Autodesk Fusion 360 part; units mm, degrees
sketch "Sketch1" plane through (0, 0, 0) normal (0, 1, 0) x (1, 0, 0)
  line L0 (-7.5, 0) -> (-20, 0)
  line L1 (-20, 0) -> (-20, 8)
  line L2 (-20, 8) -> (20, 8)
  line L3 (20, 8) -> (20, 0)
  line L4 (20, 0) -> (7.5, 0)
  arc A0 (-7.5, 0) -> (7.5, 0) centre (0, 0) ccw
  circle A1 centre (0, 0) radius 4
  dimension "d1" = 15
  dimension "d2" = 20
  dimension "d3" = 20
  dimension "d4" = 8
  dimension "d5" = 8
extrude "Extrude1" add sketch "Sketch1" along normal blind 30 contours L0 L1 L2 L3 L4 A0 | A1
extrude "Extrude2" cut sketch "Sketch1" along normal blind 15 contours A1
fillet "Fillet1" radius 3 4 edges at (-7.5, 15, 0) (7.5, 15, 0) (20, 15, 0) (-20, 15, 0)
sketch "Sketch2" plane through (0, 0, 0) normal (0, 0, 1) x (-1, 0, 0)
  line L0 (-17, 0) -> (-17, -30)
  line L1 (-17, -30) -> (-10.0623, -30)
  line L2 (-10.0623, -30) -> (-10.0623, 0)
  line L3 (-10.0623, 0) -> (-17, 0)
  circle A0 centre (14, -15) radius 1.6
  circle A1 centre (-14, -15) radius 1.6
  line L4 (10.0623, 0) -> (17, 0)
  dimension "d12" = 3.2
  dimension "d13" = 15
  dimension "d14" = 14
  dimension "d15" = 14
extrude "Extrude3" cut sketch "Sketch2" against normal through all contours A0 | A1
fillet "Fillet2" radius 3 9 edges at (-20, 30, -5.5) (-19.1213, 30, -0.8787) (-13.5312, 30, 0) (-8.2695, 30, 0.5946) (0, 30, 7.5) (8.2695, 30, 0.5946) (13.5312, 30, 0) (19.1213, 30, -0.8787) (20, 30, -5.5)
equation "d3 = d2"
equation "d15 = d14"
The model under review builds one solid part; all positions refer to its coordinate system, in mm. A direction names the side the tool comes from. Round coordinates to 2 decimals unless told otherwise and drop trailing zeros. Loops run counter-clockwise (first coordinate to the right, second up) from the corner with the lowest first, then second, coordinate; pieces in that order, holes last. Notation, with made-up numbers: (33.5, 5) - (92.5, 5) arc R3 cw to (92.5, 10) - close; hole circle Ø10 at (62, 81.5). An arc over 180 degrees is marked (long way). Use a Markdown table: item, result. Add a question column.
Q1. Add section D-D (y = 18.5). State the section outline as (x, z) points, plus the area to 3 significant figures.
Q2. Add section A-A (z = -5.5). State the section outline as (x, y) points.
Q3. The part is to be moulded in two halves that separate along X. For faces 1 (the face through (-12.4, 14.93, -3.94)), 2 (the face through (13.48, 29.1, -0.86)), 3 (the face through (-8.25, 13.69, 0.61)), say which applies: pulls with the +X half, pulls with the -X half, needs draft (parallel to the pull), parting line crosses it, or undercut.
Q4. Add section C-C (y = 3.5). State the section outline as (x, z) points.
Q5. For probe 1 along Z at (x, y) = (0, 6); probe 2 along Z at (x, y) = (6, 8.75); probe 3 along Y at (x, z) = (-14, -5.75), list the stretches that pass through material, from the lowest coordinate up.
Q6. Add section B-B (x = -14). State the section outline as (y, z) points, plus the area to 3 significant figures.
Q7. Insertion check: pin 1 Ø7.5 at (x, y) = (12.5, 9) entering from +Z; pin 2 Ø3.5 at (x, y) = (-13, 19.5) entering from +Z; pin 3 Ø5 at (y, z) = (4, 0) entering from -X. Each pin has a flat end and moves straight along its axis. Give the tip position at first contact, or say it passes through.
Q8. Machinability: for faces 4 (the face through (-0.867, 7.395, -3.905)), 5 (the face through (-13, 13, 0)), 6 (the face through (14, 13, 0)), which of the approach directions +Z, -Z, +X, -X, +Y, -Y give a long, thin tool a straight path to every point of the face, cutting with its end or side? Answer none if there is none.
Worked answers:
| question | item | result |
|---|---|---|
| 1 | outline | (-20, -8) - (20, -8) - (20, -3) arc R3 ccw to (17, 0) - (10.06, 0) arc R3 cw to (7.19, 2.14) arc R7.5 ccw to (-7.19, 2.14) arc R3 cw to (-10.06, 0) - (-17, 0) arc R3 ccw to (-20, -3) - close |
| 1 | area | 407 mm² |
| 2 | outline | (-20, 0) - (20, 0) - (20, 27) arc R3 ccw to (17, 30) - (-17, 30) arc R3 ccw to (-20, 27) - close; hole circle Ø3.2 at (-14, 15); hole circle Ø3.2 at (14, 15) |
| 3 | face 1 | undercut |
| 3 | face 2 | needs draft |
| 3 | face 3 | pulls with the -X half |
| 4 | outline | (-20, -8) - (20, -8) - (20, -3) arc R3 ccw to (17, 0) - (10.06, 0) arc R3 cw to (7.19, 2.14) arc R7.5 ccw to (-7.19, 2.14) arc R3 cw to (-10.06, 0) - (-17, 0) arc R3 ccw to (-20, -3) - close; hole circle Ø8 at (0, 0) |
| 5 | probe 1 | -8 to -4, 4 to 7.5 |
| 5 | probe 2 | -8 to 4.5 |
| 5 | probe 3 | 0 to 13.4, 16.6 to 30 |
| 6 | outline | (0, -8) - (13.4, -8) - (13.4, 0) - (0, 0) - close; (16.6, -8) - (30, -8) - (30, -3) arc R3 ccw to (27, 0) - (16.6, 0) - close |
| 6 | area | 212 mm² |
| 7 | pin 1 | z = 0.3 |
| 7 | pin 2 | z = 0 |
| 7 | pin 3 | x = -19.96 |
| 8 | face 4 | -Y |
| 8 | face 5 | +Z, -X, +Y, -Y |
| 8 | face 6 | +Z, +X, +Y, -Y |
